The listing builds one solid part. Answer for the finished solid, in the listing's coordinates (mm). A direction names the side the tool comes from. Give positions to 0.01 mm unless a question says otherwise; leave off trailing zeros. Write each loop counter-clockwise with the first axis right and the second up, starting at its lowest first coordinate (ties: lowest second). Pieces come first, ordered by that corner, then holes. Notation, with made-up numbers: M 38.5,22 L 88.5,22 A22 cw 88.5,29 Z; hole C 8,-15.75 d2. An arc over 180 degrees is marked long. Answer as a JSON object with one key per item and string values.
```python
from build123d import *

# Parameters (mm, degrees)
F0_W     = 60
F0_H     = 60
F1_DEPTH = 1.2
F3_DEPTH = 1


with BuildPart() as f1:
    # F0 (on Top) → F1 (new body)
    with BuildSketch(Plane.XY):
        Rectangle(F0_W, F0_H)
    extrude(amount=F1_DEPTH)

    # F2 (on face) → F3 (cut)
    with BuildSketch(Plane.XY.offset(1.2)):
        with BuildLine():
            Line((-22.75, 16.3925285815), (-22.75, 27.1074714185))
            ThreePointArc((-22.75, 27.1074714185), (-27.2, 21.75), (-22.75, 16.3925285815))
        make_face()
        with BuildLine():
            ThreePointArc((-16.3, 21.75), (-18.2677234458, 25.9424038451), (-22.75, 27.1074714185))
            Line((-22.75, 27.1074714185), (-22.75, 16.3925285815))
            ThreePointArc((-22.75, 16.3925285815), (-18.2677234458, 17.5575961549), (-16.3, 21.75))
        make_face()
        with BuildLine():
            Line((22.75, 16.3925285815), (22.75, 27.1074714185))
            ThreePointArc((22.75, 27.1074714185), (16.3, 21.75), (22.75, 16.3925285815))
        make_face()
        with BuildLine():
            ThreePointArc((22.75, 16.3925285815), (25.9424038451, 18.2677234458), (27.2, 21.75))
            ThreePointArc((27.2, 21.75), (25.9424038451, 25.2322765542), (22.75, 27.1074714185))
            Line((22.75, 27.1074714185), (22.75, 16.3925285815))
        make_face()
        with BuildLine():
            Line((22.75, -27.1074714185), (22.75, -16.3925285815))
            ThreePointArc((22.75, -16.3925285815), (16.3, -21.75), (22.75, -27.1074714185))
        make_face()
        with BuildLine():
            ThreePointArc((27.2, -21.75), (25.9424038451, -18.2677234458), (22.75, -16.3925285815))
            Line((22.75, -16.3925285815), (22.75, -27.1074714185))
            ThreePointArc((22.75, -27.1074714185), (25.9424038451, -25.2322765542), (27.2, -21.75))
        make_face()
        with BuildLine():
            ThreePointArc((-22.75, -16.3925285815), (-27.2, -21.75), (-22.75, -27.1074714185))
            Line((-22.75, -27.1074714185), (-22.75, -16.3925285815))
        make_face()
        with BuildLine():
            Line((-22.75, -16.3925285815), (-22.75, -27.1074714185))
            ThreePointArc((-22.75, -27.1074714185), (-18.2677234458, -25.9424038451), (-16.3, -21.75))
            ThreePointArc((-16.3, -21.75), (-18.2677234458, -17.5575961549), (-22.75, -16.3925285815))
        make_face()
    extrude(amount=-F3_DEPTH, mode=Mode.SUBTRACT)


solid = f1.part
```
1. A cutting plane is placed at A-A, the plane z = 0.55. Give the vertices of the cut face in (x, y), plus the area to 3 significant figures.
Verdict:
{"outline": "M -30,-30 L 30,-30 L 30,30 L -30,30 Z; hole C -21.75,-21.75 d10.9; hole C -21.75,21.75 d10.9; hole C 21.75,-21.75 d10.9; hole C 21.75,21.75 d10.9", "area": "3,230 mm2"}
2. The mould has two halves that part along Y. Classify faces 1 (the flat face through (0, 0, 1.2)), 2 (the flat face through (22, -22, 0.2)): released by +Y, released by -Y, zero draft, split by the parting line, or undercut.
Verdict:
{"face 1": "zero draft", "face 2": "undercut"}
3. A cutting plane is placed at B-B, the plane x = 21.75. Give the vertices of the cut face in (y, z).
Verdict:
{"outline": "M -30,0 L 30,0 L 30,1.2 L 27.2,1.2 L 27.2,0.2 L 16.3,0.2 L 16.3,1.2 L -16.3,1.2 L -16.3,0.2 L -27.2,0.2 L -27.2,1.2 L -30,1.2 Z"}
4. A flat-ended cylindrical pin translates along its axis: pin 1 (3.5 mm diameter, centred on x = 22, y = 19, fed in from +Z). Find the tip coordinate at first contact, or state that the pin passes through.
Verdict:
{"pin 1": "stops at z = 0.2"}
5. For faces 3 (the flat face through (22, 22, 0.2)), 4 (the flat face through (0, 0, 0)), determine the directions among +Z, -Z, +X, -X, +Y, -Y from which every point of the face is accessible in a straight line to the end or side of a thin tool.
Verdict:
{"face 3": "+Z", "face 4": "-Z, +X, -X, +Y, -Y"}
6. Consider line 1 along Y through (x, z) = (21.75, 0.85); line 2 along X through (y, z) = (22, 0.6); line 3 along X through (y, z) = (-26.5, 1.15). Determine where each line is inside the solid, lowest interval first.
Verdict:
{"line 1": "y = -30 to -27.2, -16.3 to 16.3, 27.2 to 30", "line 2": "x = -30 to -27.19, -16.31 to 16.31, 27.19 to 30", "line 3": "x = -30 to -24.42, -19.08 to 19.08, 24.42 to 30"}
7. A cutting plane is placed at C-C, the plane y = -23.5. Give the vertices of the cut face in (x, z).
Verdict:
{"outline": "M -30,0 L 30,0 L 30,1.2 L 26.91,1.2 L 26.91,0.2 L 16.59,0.2 L 16.59,1.2 L -16.59,1.2 L -16.59,0.2 L -26.91,0.2 L -26.91,1.2 L -30,1.2 Z"}
